from build123d import *

# Parameters (mm, degrees)
F1_DEPTH  = 50.8
F2_W      = 12.7
F2_H      = 31.75
F3_DEPTH  = 19.05
F5_DEPTH  = 12.7
F6_W      = 12.7
F6_H      = 31.75
F7_DEPTH  = 19.05
F9_DEPTH  = 12.7
F11_DEPTH = 25.4


with BuildPart() as f1:
    # F0 (on Right) → F1 (new body)
    with BuildSketch(Plane.YZ):
        Polygon((19.05, 0), (0, 0), (-19.05, 0), (-19.05, -31.75), (19.05, -31.75), align=None)
    extrude(amount=F1_DEPTH)

    # F2 (on face) → F3 (cut)
    with BuildSketch(Plane.YZ.offset(50.8)):
        with Locations((-12.7, -15.875)):
            Rectangle(F2_W, F2_H)
    extrude(amount=-F3_DEPTH, mode=Mode.SUBTRACT)

    # F4 (on face) → F5 (cut)
    with BuildSketch(Plane.XZ.offset(19.05)):
        Polygon((31.75, -31.75), (31.75, 0), (19.05, 0), align=None)
    extrude(amount=-F5_DEPTH, mode=Mode.SUBTRACT)

    # F6 (on face) → F7 (cut)
    with BuildSketch(Plane.YZ.offset(50.8)):
        with Locations((12.7, -15.875)):
            Rectangle(F6_W, F6_H)
    extrude(amount=-F7_DEPTH, mode=Mode.SUBTRACT)

    # F8 (on face) → F9 (cut)
    with BuildSketch(Plane(origin=(0, 19.05, 0), x_dir=(-1, 0, 0), z_dir=(0, 1, 0))):
        Polygon((-19.05, 0), (-31.75, 0), (-31.75, -31.75), align=None)
    extrude(amount=-F9_DEPTH, mode=Mode.SUBTRACT)

    # F10 (on face) → F11 (cut)
    with BuildSketch(Plane.XZ.offset(6.35)):
        Polygon((38.1, 0), (50.8, -31.75), (50.8, 0), align=None)
    extrude(amount=-F11_DEPTH, mode=Mode.SUBTRACT)


solid = f1.part
Could you check a few things on this model? Use its own coordinates, in mm. A direction names the side the tool comes from. Give positions to 0.01 mm unless a question says otherwise; leave off trailing zeros. Order: outer loops, then holes, each group sorted by start corner. A loop starts at its lowest first (then second) coordinate and runs counter-clockwise, first axis right, second up.
1. Suppose I cut it at C-C (y = -9.5). List the corners of the cut face in (x, z) for me, plus the area to 3 significant figures.
2. Suppose I cut it at A-A (z = -5). List the corners of the cut face in (x, y) for me.
3. I need wall thicknesses on L1, parallel to Y at x = 36, z = -12; L2, parallel to X at y = 13.5, z = -9. Which ranges of each line are inside material? Lowest first, please.
4. Suppose I cut it at B-B (x = 27.5). List the corners of the cut face in (y, z) for me (3 decimals), plus the area to 3 significant figures.
5. Suppose I cut it at D-D (y = 3.5). List the corners of the cut face in (x, z) for me, plus the area to 3 significant figures.
6. For faces 1 (the flat face through (25.31, -12.79, -15.65)), 2 (the flat face through (35, 6.35, -16)), 3 (the flat face through (19, 0, -31.75)), which set-ups out of +Z, -Z, +X, -X, +Y, -Y let a thin tool reach every point of the face, with its end or its side?
7. Will these pins go through, and if not, where does the flat tip stop? P1, Ø10, axis at y = -2.5, z = -24.5, coming from the +X side; P2, Ø1.5, axis at x = 30.5, y = 11, coming from the +Z side; P3, Ø3, axis at x = 35, z = -19.5, coming from the -Y side.
Solved:
1. outline: (0, -31.75) - (31.75, -31.75) - (19.05, 0) - (0, 0) - close
1. area: 806 mm2
2. outline: (0, -19.05) - (21.05, -19.05) - (21.05, -6.35) - (40.1, -6.35) - (40.1, 6.35) - (21.05, 6.35) - (21.05, 19.05) - (0, 19.05) - close
3. L1: y = -6.35 to 6.35
3. L2: x = 0 to 22.65
4. outline: (-19.05, -31.75) - (19.05, -31.75) - (19.05, -21.125) - (6.35, -21.125) - (6.35, 0) - (-6.35, 0) - (-6.35, -21.125) - (-19.05, -21.125) - close
4. area: 673 mm2
5. outline: (0, -31.75) - (50.8, -31.75) - (38.1, 0) - (0, 0) - close
5. area: 1,410 mm2
6. face 1: +Z, +X, -Y
6. face 2: +Z, +X, +Y
6. face 3: -Z, +X, -X, +Y, -Y
7. P1: stops at x = 49.9
7. P2: stops at z = -26.75
7. P3: stops at y = -6.35
